from build123d import *

# Parameters (mm, degrees)
SKETCH1_W           = 30
SKETCH1_H           = 30
BOSS_EXTRUDE1_DEPTH = 30
SKETCH2_R           = 10
BOSS_EXTRUDE2_DEPTH = 225
SKETCH3_W           = 30
SKETCH3_H           = 30
BOSS_EXTRUDE3_DEPTH = 50
SKETCH4_W           = 30
SKETCH4_H           = 15
CUT_EXTRUDE1_DEPTH  = 40
SKETCH5_R           = 7.5
BOSS_EXTRUDE4_DEPTH = 15
FILLET1_R           = 7.5


with BuildPart() as part:
    # Sketch1 → Boss-Extrude1 (new body)
    with BuildSketch(Plane(origin=(0, 0, 0), x_dir=(1, 0, 0), z_dir=(0, 1, 0))):
        Rectangle(SKETCH1_W, SKETCH1_H)
    extrude(amount=BOSS_EXTRUDE1_DEPTH)

    # Sketch2 → Boss-Extrude2 (add)
    with BuildSketch(Plane(origin=(0, 30, 0), x_dir=(1, 0, 0), z_dir=(0, 1, 0))):
        Circle(SKETCH2_R)
    extrude(amount=BOSS_EXTRUDE2_DEPTH)

    # Sketch3 → Boss-Extrude3 (add)
    with BuildSketch(Plane(origin=(0, 255, 0), x_dir=(1, 0, 0), z_dir=(0, 1, 0))):
        Rectangle(SKETCH3_W, SKETCH3_H)
    extrude(amount=BOSS_EXTRUDE3_DEPTH)

    # Sketch4 → Cut-Extrude1 (cut)
    with BuildSketch(Plane(origin=(0, 305, 0), x_dir=(1, 0, 0), z_dir=(0, 1, 0))):
        Rectangle(SKETCH4_W, SKETCH4_H)
    extrude(amount=-CUT_EXTRUDE1_DEPTH, mode=Mode.SUBTRACT)

    # Sketch5 → Boss-Extrude4 (add)
    with BuildSketch(Plane(origin=(0, 0, 7.5), x_dir=(-1, 0, 0), z_dir=(0, 0, -1))):
        with Locations((0, 292.5)):
            Circle(SKETCH5_R)
    extrude(amount=BOSS_EXTRUDE4_DEPTH)

    # Fillet1
    fillet1_edges = [part.edges().sort_by_distance(p)[0] for p in [
        (15, 305, 11.25),
        (-15, 305, -11.25),
        (15, 305, -11.25),
        (-15, 305, 11.25),
    ]]
    fillet(fillet1_edges, radius=FILLET1_R)


solid = part.part
Work out the finished part from the listing and answer in its coordinate system (mm). A direction names the side the tool comes from. Round coordinates to 2 decimals unless told otherwise and drop trailing zeros. Write each loop counter-clockwise with the first axis right and the second up, starting at its lowest first coordinate (ties: lowest second). Pieces come first, ordered by that corner, then holes. Notation, with made-up numbers: (64.25, 15) - (68.25, 15) arc R14 cw to (68.25, 41) - close; hole circle Ø10 at (-11, 44). An arc over 180 degrees is marked (long way). Answer in a Markdown table with one row per item. Add a question column.
1. A cutting plane is placed at C-C, the plane y = 292.5. Determine the outline of the cut face in (x, z), and give its area (3 significant figures).
2. For faces 4 (the flat face through (15, 271, 10)), 5 (the cylindrical face through (1.63, 285.18, 0.11)), determine the directions among +Z, -Z, +X, -X, +Y, -Y from which every point of the face is accessible in a straight line to the end or side of a thin tool.
3. A cutting plane is placed at A-A, the plane z = 12.5. Determine the outline of the cut face in (x, y).
4. Find the intervals of material crossed by line 1 along Y through (x, z) = (11.5, 4); line 2 along Z through (x, y) = (-1, 223.5); line 3 along Y through (x, z) = (5.5, 1.5), in increasing order. Write a range as from..to.
5. A cutting plane is placed at B-B, the plane x = 0. Determine the outline of the cut face in (y, z), and give its area (4 significant figures).
6. A cutting plane is placed at D-D, the plane x = 12.5. Determine the outline of the cut face in (y, z).
7. Given pin 1 (4 mm diameter, centred on y = 63.5, z = -3.5, fed in from +X); pin 2 (5 mm diameter, centred on x = -5, y = 142, fed in from +Z); pin 3 (4.5 mm diameter, centred on x = -4, z = -2, fed in from +Y), each flat-ended and moving along its own axis, determine where each tip first touches the part or whether it passes through.
8. The mould has two halves that part along Z. Classify faces 1 (the flat face through (0, 265, 0)), 2 (the flat face through (-15, 271, 10)), 3 (the flat face through (0, 280, -15)): +Z half, -Z half, draft (parallel to the pull), parting line (faces both ways), or undercut.
Worked out:
| question | item | result |
|---|---|---|
| 1 | outline | (-15, -15) - (15, -15) - (15, -7.5) - (7.5, -7.5) - (7.5, 7.5) - (15, 7.5) - (15, 15) - (-15, 15) - (-15, 7.5) - (-7.5, 7.5) - (-7.5, -7.5) - (-15, -7.5) - close |
| 1 | area | 675 mm^2 |
| 2 | face 4 | +Z, -Z, +X, +Y, -Y |
| 2 | face 5 | none |
| 3 | outline | (-15, 0) - (15, 0) - (15, 30) - (-15, 30) - close; (-15, 255) - (15, 255) - (15, 297.5) arc R7.5 ccw to (7.5, 305) - (-7.5, 305) arc R7.5 ccw to (-15, 297.5) - close |
| 4 | line 1 | 0..30, 255..265 |
| 4 | line 2 | -9.95..9.95 |
| 4 | line 3 | 0..265, 287.4..297.6 |
| 5 | outline | (0, -15) - (30, -15) - (30, -10) - (255, -10) - (255, -15) - (305, -15) - (305, -7.5) - (300, -7.5) - (300, 7.5) - (305, 7.5) - (305, 15) - (255, 15) - (255, 10) - (30, 10) - (30, 15) - (0, 15) - close; hole (265, -7.5) - (285, -7.5) - (285, 7.5) - (265, 7.5) - close |
| 5 | area | 6,525 mm^2 |
| 6 | outline | (0, -15) - (30, -15) - (30, 15) - (0, 15) - close; (255, -15) - (303.09, -15) - (303.09, -7.5) - (265, -7.5) - (265, 7.5) - (303.09, 7.5) - (303.09, 15) - (255, 15) - close |
| 7 | pin 1 | x = 9.89 |
| 7 | pin 2 | z = 9.68 |
| 7 | pin 3 | y = 299.79 |
| 8 | face 1 | undercut |
| 8 | face 2 | draft |
| 8 | face 3 | -Z half |
